Source: CAD feature listing. Evaluate the final solid. Frame: model axes, mm. A direction names the side the tool comes from. Coordinates: 2 decimals unless noted, no trailing zeros. Write each loop counter-clockwise with the first axis right and the second up, starting at its lowest first coordinate (ties: lowest second). Pieces come first, ordered by that corner, then holes. Notation, with made-up numbers: (69, 6.25) - (122, 6.25) arc R18 ccw to (122, 26.25) - close; hole circle Ø3 at (-20, -36.75). An arc over 180 degrees is marked (long way). One line per question, with ' | ' between items.
from build123d import *

# Parameters (mm, degrees)
F0_W     = 30
F0_H     = 5
F1_DEPTH = 35
F0_R     = 5
F2_DEPTH = 10
F0_W_2   = 10
F0_H_2   = 15
F3_DEPTH = 35
F5_DEPTH = 10.001
F7_DEPTH = 10.001


with BuildPart() as f1:
    # F0 (on Front) → F1 (new body)
    with BuildSketch(Plane.XZ):
        Polygon((-32.5, -20), (-22.5, -20), (-22.5, -15), (-22.5, -10), (-22.5, 0), (-32.5, 0), align=None)
        with Locations((-7.5, -12.5)):
            Rectangle(F0_W, F0_H)
    extrude(amount=F1_DEPTH)

    # F0 (on Front) → F2 (join)
    with BuildSketch(Plane.XZ):
        Polygon((32.5, 0), (-7.5, 20), (-32.5, 20), (-32.5, 15), (-22.5, 15), (-22.5, 0), (-22.5, -10), (7.5, -10), (7.5, -15), (-22.5, -15), (-22.5, -20), (32.5, -20), align=None)
        with Locations((17.5, -7.159092)):
            Circle(F0_R, mode=Mode.SUBTRACT)
    extrude(amount=F2_DEPTH)

    # F0 (on Front) → F3 (join)
    with BuildSketch(Plane.XZ):
        with Locations((-27.5, 7.5)):
            Rectangle(F0_W_2, F0_H_2)
    extrude(amount=F3_DEPTH)

    # F4 (on face) → F5 (cut, through all)
    with BuildSketch(Plane.XY.offset(-10)):
        Polygon((7.5, -10), (-22.5, -35), (7.5, -35), align=None)
    extrude(amount=-F5_DEPTH, mode=Mode.SUBTRACT)

    # F6 (on face) → F7 (cut, through all)
    with BuildSketch(Plane.YZ.offset(-22.5)):
        Polygon((-35, 15), (-35, 2.5), (-15, 15), align=None)
    extrude(amount=-F7_DEPTH, mode=Mode.SUBTRACT)


solid = f1.part
Item 1: Cut plane B-B on y = -21. Return loops of the section in (x, z), and give its area (4 significant figures).
Check sheet entries:
outline: (-32.5, -20) - (-22.5, -20) - (-22.5, -15) - (-5.7, -15) - (-5.7, -10) - (-22.5, -10) - (-22.5, 11.25) - (-32.5, 11.25) - close | area: 396.5 mm²
Item 2: Cut plane C-C on z = 8.5. Return loops of the section in (x, y), and give its area (3 significant figures).
Check sheet entries:
outline: (-32.5, -25.4) - (-22.5, -25.4) - (-22.5, -10) - (15.5, -10) - (15.5, 0) - (-32.5, 0) - close | area: 634 mm²
Item 3: Access query for faces 1 (the face through (-22.5, -22, -18)), 2 (the face through (-28, -12, 15)), 3 (the face through (-22.5, -22, 0)), 4 (the face through (32.5, -5, -10)), 5 (the face through (-8, 0, 0)). Directions: +Z, -Z, +X, -X, +Y, -Y. A direction counts if a zero-diameter tool reaches every point of the face in a straight line with its end or side. Return the directions, or none.
Check sheet entries:
face 1: -Z, +X, -Y | face 2: +Z, +X, -X, -Y | face 3: +Z, +X, -Y | face 4: +Z, -Z, +X, +Y, -Y | face 5: +Z, -Z, +X, -X, +Y
Item 4: Cut plane A-A on x = 17.5. Return loops of the section in (y, z).
Check sheet entries:
outline: (-10, -20) - (0, -20) - (0, -12.16) - (-10, -12.16) - close; (-10, -2.16) - (0, -2.16) - (0, 7.5) - (-10, 7.5) - close
Item 5: Pin query (flat end, axial travel): pin 1 Ø10 at (x, y) = (6.5, -14) entering from +Z; pin 2 Ø3 at (x, z) = (-26, 5) entering from -Y; pin 3 Ø10 at (x, y) = (-8, -28) entering from -Z. Return the tip coordinate at first contact, or that it passes through.
Check sheet entries:
pin 1: z = 14.5 | pin 2: y = -33.4 | pin 3: z = -15
Item 6: Ray query, line 1 along Z through (x, y) = (17.5, -5.75); line 2 along Y through (x, z) = (-13.5, -2.5); line 3 along X through (y, z) = (-15, -6.5). Return the intervals inside material, ascending. Write a range as [from, to].
Check sheet entries:
line 1: [-20, -12.16], [-2.16, 7.5] | line 2: [-10, 0] | line 3: [-32.5, -22.5]
Item 7: Cut plane D-D on x = -3. Return loops of the section in (y, z).
Check sheet entries:
outline: (-18.75, -15) - (-10, -15) - (-10, -20) - (0, -20) - (0, 17.75) - (-10, 17.75) - (-10, -10) - (-18.75, -10) - close
Item 8: Mould query, pull axis X, two halves, no side actions, for faces 6 (the face through (16.85, -4.93, -2.2)), 7 (the face through (-32.5, -17, -5)), 8 (the face through (0, -10, 0)), 9 (the face through (-7.29, -22.325, -12.465)). Classes: pulls with the +X half, pulls with the -X half, needs draft (parallel to the pull), parting line crosses it, or undercut.
Check sheet entries:
face 6: undercut | face 7: pulls with the -X half | face 8: needs draft | face 9: pulls with the +X half
